CAD build for the part. Positions are in the model's coordinates, mm. A direction names the side the tool comes from. Give positions to 0.01 mm unless a question says otherwise; leave off trailing zeros. Loops run counter-clockwise (first coordinate to the right, second up) from the corner with the lowest first, then second, coordinate; pieces in that order, holes last.
```python
from build123d import *

# Parameters (mm, degrees)
SKETCH1_W               = 330.2
SKETCH1_H               = 457.2
BOSS_EXTRUDE1_DEPTH     = 203.2
CUT_EXTRUDE1_DEPTH      = 115.316
CUT_EXTRUDE1_DEPTH_BACK = 294.386
SKETCH2_W               = 254
SKETCH2_H               = 152.4
SKETCH3_R               = 12.7
BOSS_EXTRUDE2_DEPTH     = 25.4


with BuildPart() as part:
    # Sketch1 → Boss-Extrude1 (new body)
    with BuildSketch(Plane.XY):
        with Locations((165.1, 228.6)):
            Rectangle(SKETCH1_W, SKETCH1_H)
    extrude(amount=BOSS_EXTRUDE1_DEPTH)

    # Sketch2 → Cut-Extrude1 (cut, two sides: drawn at the far end of the back side and taken through both)
    with BuildSketch(Plane.XY.offset(203.2).offset(-CUT_EXTRUDE1_DEPTH_BACK)):
        with Locations((165.1, 76.2)):
            Rectangle(SKETCH2_W, SKETCH2_H)
    extrude(amount=CUT_EXTRUDE1_DEPTH + CUT_EXTRUDE1_DEPTH_BACK, mode=Mode.SUBTRACT)

    # Sketch3 → Boss-Extrude2 (add)
    with BuildSketch(Plane.ZY.offset(-292.1)):
        with Locations(Location((101.6, 12.7, 0), (0, 0, 270))):
            Circle(SKETCH3_R)
    boss_extrude2 = extrude(amount=BOSS_EXTRUDE2_DEPTH)

    # Mirror1: Boss-Extrude2 across plane
    add(boss_extrude2.mirror(Plane.ZY.offset(-165.1)))


solid = part.part
```
1. Tool access for faces 5 (the face through (311, 0, 100)), 6 (the face through (279.578, 14.353, 114.192)), 7 (the face through (266.7, 13, 102)): list every direction of +Z, -Z, +X, -X, +Y, -Y with a clear straight run to the whole face (end or side of a thin tool).
Responses:
face 5: +Z, -Z, +X, -X, -Y
face 6: none
face 7: +Z, -Z, -Y
2. Saw through at B-B, the plane z = 138.5. List the corners of the cut face in (x, y), and give its area (3 significant figures).
Responses:
outline: (0, 0) - (38.1, 0) - (38.1, 152.4) - (292.1, 152.4) - (292.1, 0) - (330.2, 0) - (330.2, 457.2) - (0, 457.2) - close
area: 112,000 mm2
3. Saw through at C-C, the plane y = 60.5. List the corners of the cut face in (x, z).
Responses:
outline: (0, 0) - (38.1, 0) - (38.1, 203.2) - (0, 203.2) - close; (292.1, 0) - (330.2, 0) - (330.2, 203.2) - (292.1, 203.2) - close
4. Pull direction X, two halves, no side cores. Call faces 1 (the face through (163, 283, 203.2)), 2 (the face through (0, 225, 100)), 3 (the face through (38.1, 75, 100)), 4 (the face through (292.1, 75, 100)): released by +X, released by -X, zero draft, split by the parting line, or undercut.
Responses:
face 1: zero draft
face 2: released by -X
face 3: undercut
face 4: undercut
5. Probe line 1 along X through (y, z) = (95.5, 190.5); line 2 along Y through (x, z) = (97, 19); line 3 along Y through (x, z) = (40, 112.5). List the from-to ranges inside material, lowest first.
Responses:
line 1: x = 0 to 38.1, 292.1 to 330.2
line 2: y = 152.4 to 457.2
line 3: y = 6.18 to 19.22, 152.4 to 457.2
6. Drop flat-ended pins along their axis: pin 1 (3 mm diameter, centred on y = 352.5, z = 132, fed in from -X); pin 2 (5 mm diameter, centred on x = 281.5, z = 122, fed in from -Y). Give the stop position or say it passes through.
Responses:
pin 1: stops at x = 0
pin 2: stops at y = 152.4
7. Saw through at A-A, the plane y = 12.7. List the corners of the cut face in (x, z), and give its area (3 significant figures).
Responses:
outline: (0, 0) - (38.1, 0) - (38.1, 88.9) - (63.5, 88.9) - (63.5, 114.3) - (38.1, 114.3) - (38.1, 203.2) - (0, 203.2) - close; (266.7, 88.9) - (292.1, 88.9) - (292.1, 0) - (330.2, 0) - (330.2, 203.2) - (292.1, 203.2) - (292.1, 114.3) - (266.7, 114.3) - close
area: 16,800 mm2
8. Saw through at D-D, the plane x = 86. List the corners of the cut face in (y, z), and give its area (3 significant figures).
Responses:
outline: (152.4, 0) - (457.2, 0) - (457.2, 203.2) - (152.4, 203.2) - close
area: 61,900 mm2
